```python
from build123d import *

# Parameters (mm, degrees)
SKETCH1_R           = 6.25
BOSS_EXTRUDE1_DEPTH = 7
BOSS_EXTRUDE2_DEPTH = 7
CIRPATTERN1_COUNT   = 12
CUT_EXTRUDE1_DEPTH  = 7


with BuildPart() as part:
    # Sketch1 → Boss-Extrude1 (new body)
    with BuildSketch(Plane.XY):
        with Locations(Location((0, 0, 0), (0, 0, 180))):
            Circle(SKETCH1_R)
    extrude(amount=BOSS_EXTRUDE1_DEPTH)

    # Sketch3 → Boss-Extrude2 (add)
    with BuildSketch(Plane.XY):
        Polygon((-0.8, 7.9), (0.8, 7.9), (1.3, 5.7), (-1.3, 5.7), align=None)
    boss_extrude2 = extrude(amount=BOSS_EXTRUDE2_DEPTH)

    # CirPattern1: Boss-Extrude2 ×12 about axis
    cirpattern1_axis = Axis((0, 0.185968122, 0), (0, 0, 1))
    for i in range(1, CIRPATTERN1_COUNT):
        add(boss_extrude2.rotate(cirpattern1_axis, i * 360 / CIRPATTERN1_COUNT))

    # Sketch4 → Cut-Extrude1 (cut)
    with BuildSketch(Plane.XY):
        with BuildLine():
            Line((1.9, 3.405877273), (1.9, -3.405877273))
            ThreePointArc((1.9, -3.405877273), (-3.9, 0), (1.9, 3.405877273))
        make_face()
    extrude(amount=CUT_EXTRUDE1_DEPTH, mode=Mode.SUBTRACT)


solid = part.part
```
For this review, take the finished solid that the model builds, in its own axes (mm). A direction names the side the tool comes from. Round coordinates to 2 decimals unless told otherwise and drop trailing zeros. Write each loop counter-clockwise with the first axis right and the second up, starting at its lowest first coordinate (ties: lowest second). Pieces come first, ordered by that corner, then holes. Notation, with made-up numbers: (77, 50.5) - (131, 50.5) arc R31 ccw to (131, 83.5) - close; hole circle Ø5 at (19, 63.25). An arc over 180 degrees is marked (long way). Write each question's results on one line, items separated by ' | '.
Item 1: For pin 1 (1.5 mm diameter, centred on x = 2, z = 2.5, fed in from +Y), flat-tipped, find the tip position at first contact; note if it passes through.
Calculated:
pin 1: stops at y = 6.82
Item 2: Take a section at B-B on x = 0. State the section outline as (y, z) points, then the cut area to 3 significant figures.
Calculated:
outline: (-7.53, 0) - (-3.9, 0) - (-3.9, 7) - (-7.53, 7) - close; (3.9, 0) - (7.9, 0) - (7.9, 7) - (3.9, 7) - close | area: 53.4 mm^2
Item 3: Take a section at A-A on y = 0. State the section outline as (x, z) points.
Calculated:
outline: (-7.71, 0) - (-3.9, 0) - (-3.9, 7) - (-7.71, 7) - close; (1.9, 0) - (7.71, 0) - (7.71, 7) - (1.9, 7) - close
Item 4: For faces 1 (the face through (1.9, 0, 3)), 2 (the face through (2.542, 6.595, 3.451)), 3 (the face through (6.51, -2.45, 3.45)), 4 (the face through (-6.52, -2.46, 3.45)), 5 (the face through (2.69, -6.38, 3.45)), list the 3-axis set-ups (+Z, -Z, +X, -X, +Y, -Y) from which the entire face can be reached by the end or side of a thin tool; tool diameter is ignored.
Calculated:
face 1: +Z, -Z | face 2: +Z, -Z, +Y | face 3: +Z, -Z, +X | face 4: +Z, -Z, -X | face 5: +Z, -Z, -Y
Item 5: Take a section at C-C on x = 3.5. State the section outline as (y, z) points.
Calculated:
outline: (-6.7, 0) - (7.07, 0) - (7.07, 7) - (-6.7, 7) - close
Item 6: To check wall thickness, follow line 1 along Y through (x, z) = (0, 4); line 2 along X through (y, z) = (0, 3.75); line 3 along Y through (x, z) = (0.75, 4). State the ranges of each line that lie inside material, in increasing order. Write a range as from..to.
Calculated:
line 1: y = -7.53..-3.9, 3.9..7.9 | line 2: x = -7.71..-3.9, 1.9..7.71 | line 3: y = -7.53..-3.83, 3.83..7.9
Item 7: Take a section at D-D on y = -5.25. State the section outline as (x, z) points, then the cut area to 3 significant figures.
Calculated:
outline: (-4.29, 0) - (4.29, 0) - (4.29, 7) - (-4.29, 7) - close | area: 60.0 mm^2
